```python
from build123d import *

# Parameters (mm, degrees)
SKETCH1_W                        = 44.45
SKETCH1_H                        = 44.45
SKETCH1_W_2                      = 38.1
SKETCH1_H_2                      = 38.1
BOSS_EXTRUDE1_DEPTH              = 355.6
BOSS_EXTRUDE1_DEPTH_BACK         = 355.6
F_17_64_0_26563_DIAMETER_HOLE1_D = 6.747002


with BuildPart() as part:
    # Sketch1 → Boss-Extrude1 (new body, two sides)
    with BuildSketch(Plane(origin=(0, 0, 0), x_dir=(0, 0, -1), z_dir=(1, 0, 0))) as boss_extrude1_sk:
        Rectangle(SKETCH1_W, SKETCH1_H)
        Rectangle(SKETCH1_W_2, SKETCH1_H_2, mode=Mode.SUBTRACT)
    extrude(amount=BOSS_EXTRUDE1_DEPTH)
    extrude(boss_extrude1_sk.sketch, amount=-BOSS_EXTRUDE1_DEPTH_BACK)

    # 17/64 (0.26563) Diameter Hole1 (through all)
    with Locations(Plane.XY.offset(22.225)):
        with Locations((-117.475, 0), (117.475, 0)):
            Hole(F_17_64_0_26563_DIAMETER_HOLE1_D / 2)


solid = part.part
```
Could you check a few things on this model? Use its own coordinates, in mm. A direction names the side the tool comes from. Round coordinates to 2 decimals unless told otherwise and drop trailing zeros. Write each loop counter-clockwise with the first axis right and the second up, starting at its lowest first coordinate (ties: lowest second). Pieces come first, ordered by that corner, then holes. Notation, with made-up numbers: M 61,31 L 69,31 A23 ccw 69,50 Z; hole C 16.25,-37 d3. An arc over 180 degrees is marked long. Write each question's results on one line, items separated by ' | '. Start each with the question number.
1. On a 3-axis mill with a long thin cutter (end or side, diameter ignored), from which of +Z, -Z, +X, -X, +Y, -Y can I reach the whole of each face in a straight line? I mean faces 1 (the face through (355.6, 0.3, -19.4)), 2 (the face through (5, 0, -19.05)). Say none if no direction works.
2. Thinking about a two-plate mould opening in Z: for faces 3 (the face through (5, 0, 22.225)), 4 (the face through (5, -19.05, 0)), 5 (the face through (-355.6, 0.3, -19.4)), which applies, +Z half, -Z half, draft (parallel to the pull), parting line (faces both ways), or undercut?
3. I need wall thicknesses on L1, parallel to Z at x = -8.5, y = 11.5 (3 decimals). Which ranges of the line are inside material? Lowest first, please. Write a range as from..to.
4. Imagine slicing it at A-A on z = -8. List the corners of the cut face in (x, y) for me (3 decimals).
5. I'm going to push a flat-ended pin straight in: pin 1 Ø4 at (x, y) = (117.475, 0) entering from +Z. Where does the tip first touch, or does it pass through?
6. Imagine slicing it at B-B on x = 208. List the corners of the cut face in (y, z) for me (3 decimals).
Result sheet:
1) face 1: +Z, -Z, +X, +Y, -Y | face 2: +X, -X
2) face 3: +Z half | face 4: undercut | face 5: draft
3) L1: z = -22.225..-19.05, 19.05..22.225
4) outline: M -355.6,-22.225 L 355.6,-22.225 L 355.6,-19.05 L -355.6,-19.05 Z; M -355.6,19.05 L 355.6,19.05 L 355.6,22.225 L -355.6,22.225 Z
5) pin 1: passes through
6) outline: M -22.225,-22.225 L 22.225,-22.225 L 22.225,22.225 L -22.225,22.225 Z; hole M -19.05,-19.05 L 19.05,-19.05 L 19.05,19.05 L -19.05,19.05 Z
